```python
from build123d import *

# Parameters (mm, degrees)
BOSS_EXTRU_1_DEPTH                          = 2
FRAISAGE_POUR_VIS_T_TE_FRAIS_E_M31_AT_COUNT = 2
FRAISAGE_POUR_VIS_T_TE_FRAIS_E_M31_AT_PITCH = 71.69


with BuildPart() as part:
    # Esquisse1 → Boss.-Extru.1 (new body)
    with BuildSketch(Plane.XY):
        with BuildLine():
            Line((-4.7, 69.04), (-4.7, 65.74))
            Line((-4.7, 65.74), (-13, 65.74))
            ThreePointArc((-13, 65.74), (-19.151828996, 63.191828996), (-21.7, 57.04))
            Line((-21.7, 57.04), (-21.7, 9.35))
            ThreePointArc((-21.7, 9.35), (-19.151828996, 3.198171004), (-13, 0.65))
            Line((-13, 0.65), (-4.7, 0.65))
            Line((-4.7, 0.65), (-4.7, -2.65))
            ThreePointArc((-4.7, -2.65), (0, -7.35), (4.7, -2.65))
            Line((4.7, -2.65), (4.7, 0.65))
            Line((4.7, 0.65), (13, 0.65))
            ThreePointArc((13, 0.65), (19.151828996, 3.198171004), (21.7, 9.35))
            Line((21.7, 9.35), (21.7, 57.04))
            ThreePointArc((21.7, 57.04), (19.151828996, 63.191828996), (13, 65.74))
            Line((13, 65.74), (4.7, 65.74))
            Line((4.7, 65.74), (4.7, 69.04))
            ThreePointArc((4.7, 69.04), (0, 73.74), (-4.7, 69.04))
        make_face()
    extrude(amount=BOSS_EXTRU_1_DEPTH)

    # Esquisse4 → Fraisage pour vis à tête fraisée M31 (revolve, cut)
    with BuildSketch(Plane(origin=(0, 69.04, 2), x_dir=(0, -1, 0), z_dir=(1, 0, 0))):
        Polygon((0, 0), (0, 2), (1.7, 2), (1.7, 1.45), (3.15, 0), align=None)
    fraisage_pour_vis_t_te_frais_e_m31 = revolve(axis=Axis((0, 69.04, 8.35), (0, 0, -1)), mode=Mode.SUBTRACT)

    # Fraisage pour vis à tête fraisée M31 at: Fraisage pour vis à tête fraisée M31 ×2
    with Locations(*[(0, -i * FRAISAGE_POUR_VIS_T_TE_FRAIS_E_M31_AT_PITCH, 0) for i in range(1, FRAISAGE_POUR_VIS_T_TE_FRAIS_E_M31_AT_COUNT)]):
        add(fraisage_pour_vis_t_te_frais_e_m31, mode=Mode.SUBTRACT)


solid = part.part
```
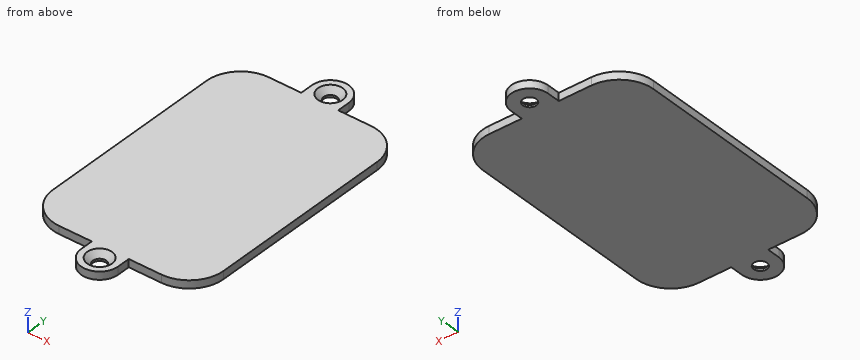
For this review, take the finished solid that the model builds, in its own axes (mm). Give positions to 0.01 mm unless a question says otherwise; leave off trailing zeros. Write each loop counter-clockwise with the first axis right and the second up, starting at its lowest first coordinate (ties: lowest second). Pieces come first, ordered by that corner, then holes. Notation, with made-up numbers: M 82.25,-25 L 94.25,-25 A29 cw 94.25,-5 Z; hole C 6.5,57.25 d8. An arc over 180 degrees is marked long. Answer as CSV lines item,"result".
1. Consider section B-B, the plane x = 0. Write out the cut boundary in (y, z), then the cut area to 3 significant figures.
Findings:
outline,"M -7.35,0 L -4.35,0 L -4.35,0.55 L -5.8,2 L -7.35,2 Z; M -0.95,0 L 67.34,0 L 67.34,0.55 L 65.89,2 L 0.5,2 L -0.95,0.55 Z; M 70.74,0 L 73.74,0 L 73.74,2 L 72.19,2 L 70.74,0.55 Z"
area,"144 mm2"
2. For pin 1 (2 mm diameter, centred on x = -3, y = 51.5, fed in from -Z); pin 2 (1 mm diameter, centred on x = 8.5, z = 1, fed in from +Y); pin 3 (1 mm diameter, centred on x = 8.5, z = 0.5, fed in from -Y); pin 4 (1 mm diameter, centred on y = -1, z = 1, fed in from +X), all flat-tipped, find the tip position at first contact; note any pin that passes through.
Findings:
pin 1,"stops at z = 0"
pin 2,"stops at y = 65.74"
pin 3,"stops at y = 0.65"
pin 4,"stops at x = 4.7"
3. Consider section D-D, the plane x = 16.5. Write out the cut boundary in (y, z), then the cut area to 3 significant figures.
Findings:
outline,"M 1.39,0 L 65,0 L 65,2 L 1.39,2 Z"
area,"127 mm2"
4. Wall thickness on line 1 (Y direction, x = 0, z = 0.25); line 2 (Y direction, x = -1.5, z = 0.85); line 3 (X direction, y = 69.04, z = 0.3): over which ranges is each line inside the solid? List them lowest first.
Findings:
line 1,"y = -7.35 to -4.35, -0.95 to 67.34, 70.74 to 73.74"
line 2,"y = -7.1 to -3.97, -1.33 to 67.72, 70.36 to 73.49"
line 3,"x = -4.7 to -1.7, 1.7 to 4.7"
5. Consider section C-C, the plane x = -10.5. Write out the cut boundary in (y, z), then the cut area to 3 significant figures.
Findings:
outline,"M 0.65,0 L 65.74,0 L 65.74,2 L 0.65,2 Z"
area,"130 mm2"
6. Consider section A-A, the plane z = 1.25. Write out the cut boundary in (x, y).
Findings:
outline,"M -21.7,9.35 A8.7 ccw -13,0.65 L -4.7,0.65 L -4.7,-2.65 A4.7 ccw 4.7,-2.65 L 4.7,0.65 L 13,0.65 A8.7 ccw 21.7,9.35 L 21.7,57.04 A8.7 ccw 13,65.74 L 4.7,65.74 L 4.7,69.04 A4.7 ccw -4.7,69.04 L -4.7,65.74 L -13,65.74 A8.7 ccw -21.7,57.04 Z; hole C 0,-2.65 d4.8; hole C 0,69.04 d4.8"
